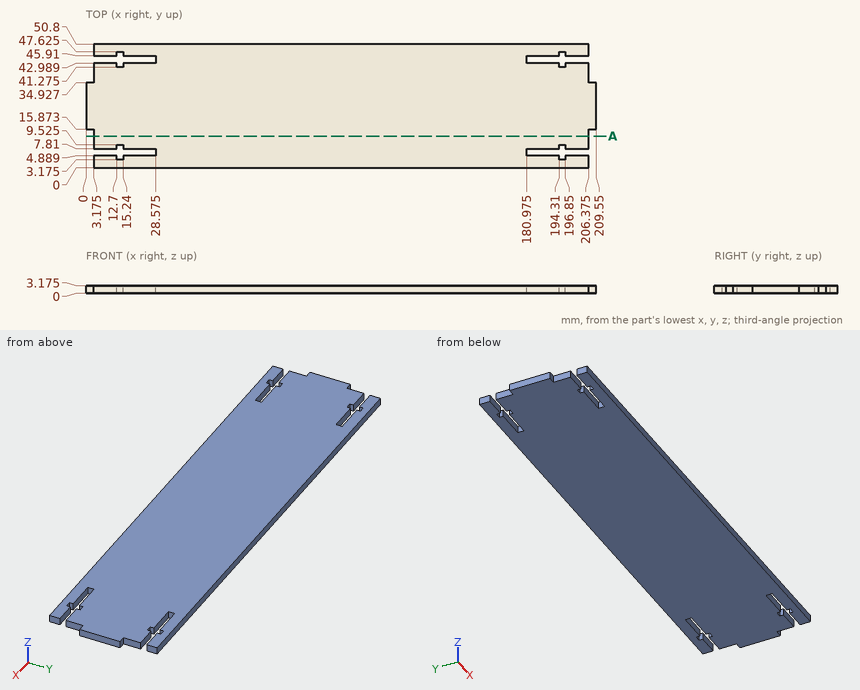
Input: dimensioned drawing with shaded views. Units: mm. Origin: part minimum x, y, z. Give positions to 0.01 mm unless a question says otherwise; leave off trailing zeros. Write each loop counter-clockwise with the first axis right and the second up, starting at its lowest first coordinate (ties: lowest second). Pieces come first, ordered by that corner, then holes.
1. First-contact query: pin 1 (1.9 mm diameter, centred on y = 8.5, z = 2, fed in from +X) (1 decimal); pin 2 (1.4 mm diameter, centred on y = 47, z = 1.5, fed in from -X) (1 decimal); pin 3 (1.5 mm diameter, centred on y = 6, z = 1, fed in from -X) (1 decimal). Flat tips, straight axial feed; report the tip coordinate or a pass-through.
2. Material intervals for line 1 along Y through (x, z) = (12, 2.7); line 2 along Y through (x, z) = (196, 0.3) (1 decimal); line 3 along X through (y, z) = (10.5, 3.05) (1 decimal), sorted ascending.
3. Section query A-A (y = 13). Return the cut outline in (x, z) (1 decimal).
Output values:
1. pin 1: stops at x = 206.4
1. pin 2: stops at x = 3.2
1. pin 3: stops at x = 28.6
2. line 1: y = 0 to 4.89, 7.81 to 42.99, 45.91 to 50.8
2. line 2: y = 0 to 3.2, 9.5 to 41.3, 47.6 to 50.8
2. line 3: x = 3.2 to 206.4
3. outline: (3.2, 0) - (206.4, 0) - (206.4, 3.2) - (3.2, 3.2) - close
